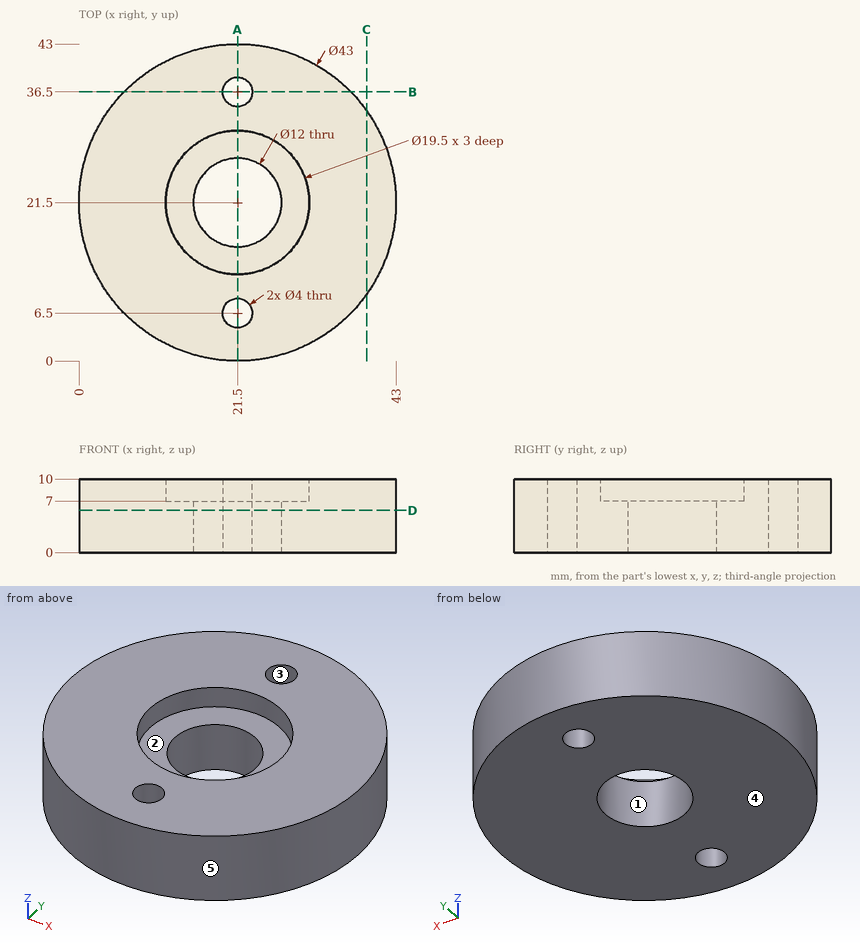
Here's the drawing with two shaded views (mm, measured from the low corner). I have some questions. A direction names the side the tool comes from. Round coordinates to 2 decimals unless told otherwise and drop trailing zeros. Write each loop counter-clockwise with the first axis right and the second up, starting at its lowest first coordinate (ties: lowest second). Pieces come first, ordered by that corner, then holes. Notation, with made-up numbers: M 27,63 L 64,63 A19 ccw 64,90 Z; hole C 7,11 d8. An arc over 180 degrees is marked long. Answer in a Markdown table with one row per item. Add a question column.
Q1. Imagine slicing it at D-D (z = 5.75). Please give me the cut outline in (x, y), then the cut area to 3 significant figures.
Q2. Will these pins go through, and if not, where does the flat tip stop? pin 1 Ø3.5 at (x, y) = (21.5, 6.5) entering from +Z; pin 2 Ø1.5 at (y, z) = (29.5, 1.5) entering from -X; pin 3 Ø6 at (x, z) = (6.5, 3.5) entering from +Y.
Q3. If we mould it in two halves opening along X, with no side actions, what happens to the marked faces 3, 4 and 5? For each: +X half, -X half, draft (parallel to the pull), parting line (faces both ways), or undercut.
Q4. Imagine slicing it at C-C (x = 39). Please give me the cut outline in (y, z).
Q5. If I drill on line 1 (Y direction, x = 21.5, z = 2.75); line 2 (Y direction, x = 21, z = 5.25); line 3 (X direction, y = 6.5, z = 7.5), over which ranges is the centre line in solid material (lowest first)? Write a range as from..to.
Q6. On a 3-axis mill with a long thin cutter (end or side, diameter ignored), from which of +Z, -Z, +X, -X, +Y, -Y can I reach the whole of each face in a straight line? I mean the marked faces 1 and 2. Say none if no direction works.
Q7. Imagine slicing it at A-A (x = 21.5). Please give me the cut outline in (y, z), then the cut area to 4 significant figures.
Q8. Imagine slicing it at B-B (y = 36.5). Please give me the cut outline in (x, z).
Values:
| question | item | result |
|---|---|---|
| 1 | outline | C 21.5,21.5 d43; hole C 21.5,21.5 d12; hole C 21.5,6.5 d4; hole C 21.5,36.5 d4 |
| 1 | area | 1,310 mm^2 |
| 2 | pin 1 | through |
| 2 | pin 2 | x = 1.26 |
| 2 | pin 3 | y = 39.34 |
| 3 | face 3 | undercut |
| 3 | face 4 | draft |
| 3 | face 5 | parting line |
| 4 | outline | M 9.01,0 L 33.99,0 L 33.99,10 L 9.01,10 Z |
| 5 | line 1 | 0..4.5, 8.5..15.5, 27.5..34.5, 38.5..43 |
| 5 | line 2 | 0.01..4.56, 8.44..15.52, 27.48..34.56, 38.44..42.99 |
| 5 | line 3 | 6.1..19.5, 23.5..36.9 |
| 6 | face 1 | +Z, -Z |
| 6 | face 2 | +Z |
| 7 | outline | M 0,0 L 4.5,0 L 4.5,10 L 0,10 Z; M 8.5,0 L 15.5,0 L 15.5,7 L 11.75,7 L 11.75,10 L 8.5,10 Z; M 27.5,0 L 34.5,0 L 34.5,10 L 31.25,10 L 31.25,7 L 27.5,7 Z; M 38.5,0 L 43,0 L 43,10 L 38.5,10 Z |
| 7 | area | 207.5 mm^2 |
| 8 | outline | M 6.1,0 L 19.5,0 L 19.5,10 L 6.1,10 Z; M 23.5,0 L 36.9,0 L 36.9,10 L 23.5,10 Z |
